Build history of the part. All positions in model axes, mm. A direction names the side the tool comes from. Round coordinates to 2 decimals unless told otherwise and drop trailing zeros. Write each loop counter-clockwise with the first axis right and the second up, starting at its lowest first coordinate (ties: lowest second). Pieces come first, ordered by that corner, then holes. Notation, with made-up numbers: M 7,70.25 L 56,70.25 A11 cw 56,91.25 Z; hole C 77,29 d6. An arc over 180 degrees is marked long. Write item = value, one per line.
from build123d import *

# Parameters (mm, degrees)
BOSS_EXTRUDE1_DEPTH = 50
CUT_EXTRUDE1_DEPTH  = 11
BOSS_EXTRUDE2_DEPTH = 50


with BuildPart() as part:
    # Sketch1 → Boss-Extrude1 (new body)
    with BuildSketch(Plane(origin=(0, 0, 0), x_dir=(0, 0, -1), z_dir=(1, 0, 0))):
        Polygon((-28.922236088, -13.479594195), (-28.922236088, 1.520405805), (-20.922236088, 1.520405805), (-20.922236088, -5.479594195), align=None)
    extrude(amount=BOSS_EXTRUDE1_DEPTH)

    # Sketch2 → Cut-Extrude1 (cut)
    with BuildSketch(Plane(origin=(50, 0, 0), x_dir=(0, 0, -1), z_dir=(1, 0, 0))):
        Polygon((-20.922236088, 1.520405805), (-26.922236088, 1.520405805), (-26.922236088, -11.479594195), (-20.922236088, -5.479594195), align=None)
    cut_extrude1 = extrude(amount=-CUT_EXTRUDE1_DEPTH, mode=Mode.SUBTRACT)

    # Mirror1: Cut-Extrude1 across plane
    add(cut_extrude1.mirror(Plane(origin=(25, 0, 0), x_dir=(0, 0, 1), z_dir=(1, 0, 0))), mode=Mode.SUBTRACT)

    # Sketch3 → Boss-Extrude2 (add, through all)
    with BuildSketch(Plane(origin=(50, 0, 0), x_dir=(0, 0, -1), z_dir=(1, 0, 0))):
        Polygon((-28.922236088, -13.479594195), (-31.735625087, -16.337129199), (-28.922236088, -11.464196511), align=None)
    extrude(amount=-BOSS_EXTRUDE2_DEPTH)


solid = part.part
1. Flat gauge pins, fed straight in: pin 1 (2 mm diameter, centred on x = 21, y = -13.5, fed in from +Z); pin 2 (4 mm diameter, centred on x = 31.5, y = -6.5, fed in from +Z); pin 3 (1.8 mm diameter, centred on y = -3, z = 24.5, fed in from -X). Where does each tip first touch, or does it go through?
Responses:
pin_1 = 30.67
pin_2 = 28.92
pin_3 = 11
2. Probe probe 1 along Z at (x, y) = (40, -2.5); probe 2 along X at (y, z) = (-5.75, 23.25); probe 3 along Z at (x, y) = (36, -2.5). List the from-to ranges inside material, lowest first.
Responses:
probe_1 = 26.92 to 28.92
probe_2 = 11 to 39
probe_3 = 20.92 to 28.92
3. Band-saw the part on C-C (z = 23.5). List the corners of the cut face in (x, y).
Responses:
outline = M 11,-8.06 L 39,-8.06 L 39,1.52 L 11,1.52 Z
4. Band-saw the part on B-B (x = 41.5). List the corners of the cut face in (y, z).
Responses:
outline = M -16.34,31.74 L -13.48,28.92 L -11.48,26.92 L 1.52,26.92 L 1.52,28.92 L -11.46,28.92 Z
5. Band-saw the part on A-A (y = -3). List the corners of the cut face in (x, z), plus the area to 3 significant figures.
Responses:
outline = M 0,26.92 L 11,26.92 L 11,20.92 L 39,20.92 L 39,26.92 L 50,26.92 L 50,28.92 L 0,28.92 Z
area = 268 mm²
6. Band-saw the part on D-D (x = 17.5). List the corners of the cut face in (y, z).
Responses:
outline = M -16.34,31.74 L -13.48,28.92 L -5.48,20.92 L 1.52,20.92 L 1.52,28.92 L -11.46,28.92 Z
7. Tool access for faces 1 (the face through (25, -5, 28.922)), 2 (the face through (11, -3, 24)), 3 (the face through (39, -3, 24)), 4 (the face through (0, -7, 28)): list every direction of +Z, -Z, +X, -X, +Y, -Y with a clear straight run to the whole face (end or side of a thin tool).
Responses:
face_1 = +Z, +X, -X, +Y
face_2 = -Z, -X, +Y, -Y
face_3 = -Z, +X, +Y, -Y
face_4 = +Z, -Z, -X, +Y, -Y
